The listing builds one solid part. Answer for the finished solid, in the listing's coordinates (mm). A direction names the side the tool comes from. Coordinates: 2 decimals unless noted, no trailing zeros. Return JSON: item names as keys, results as strings. Group by question number.
1. Which of the six approach directions +Z, -Z, +X, -X, +Y, -Y give full straight-line access (tool end or side, diameter ignored) to faces 4 (the face through (-22.23, 10.37, -10.32)), 5 (the face through (-33.142, 10.018, -8.724))?
2. Each of these flat-tipped pins is pushed along its axis until it touches: P1, Ø1.5, axis at y = 6.5, z = -7.5, coming from the +X side; P2, Ø4.5, axis at x = -26.99, y = 10.16, coming from the +Z side; P3, Ø12.5, axis at x = -17.46, z = 0, coming from the -Y side; P4, Ø1, axis at x = -7.5, z = -9, coming from the -Y side. Where does it stop, or does it pass through?
3. Section A-A (z = 0) is taken. State how many separate pieces and enclosed holes the cut face has, and give its area (3 significant figures).
4. Find the intervals of material crossed by line 1 along X through (y, z) = (6, -10); line 2 along Z through (x, y) = (-28, 13.75); line 3 along X through (y, z) = (10.16, -10.7) (3 decimals), in increasing order.
5. The mould has two halves that part along Z. Classify faces 1 (the face through (-10, 8, -7.874)), 2 (the face through (-34.925, 10, 3)), 3 (the face through (-22.22, 10.15, 0.21)): pulls with the +Z half, pulls with the -Z half, needs draft (parallel to the pull), parting line crosses it, or undercut.
```python
from build123d import *

# Parameters (mm, degrees)
BOSS_EXTRUDE1_DEPTH                             = 10.16
BOSS_EXTRUDE1_DEPTH_BACK                        = 12.7
SKETCH2_W                                       = 34.925
SKETCH2_H                                       = 20.32
SKETCH2_R                                       = 2.4892
SKETCH3_R                                       = 4.7625
CUT_EXTRUDE1_DEPTH                              = 43.35502361
CBORE_FOR_10_SOCKET_HEAD_CAP_SCREW1_D           = 4.9784
CBORE_FOR_10_SOCKET_HEAD_CAP_SCREW1_CBORE_D     = 9.525
CBORE_FOR_10_SOCKET_HEAD_CAP_SCREW1_CBORE_DEPTH = 4.826
FILLET1_R                                       = 9.525


with BuildPart() as part:
    # Sketch2 → Boss-Extrude1 (new, two sides: drawn at the far end of the back side and taken through both)
    with BuildSketch(Plane.XY.offset(-BOSS_EXTRUDE1_DEPTH_BACK)):
        with Locations((-17.4625, 10.16)):
            Rectangle(SKETCH2_W, SKETCH2_H)
        with Locations((-7.9375, 10.16)):
            Circle(SKETCH2_R, mode=Mode.SUBTRACT)
        with Locations((-26.9875, 10.16)):
            Circle(SKETCH2_R, mode=Mode.SUBTRACT)
    extrude(amount=BOSS_EXTRUDE1_DEPTH + BOSS_EXTRUDE1_DEPTH_BACK)

    # Sketch3 → Cut-Extrude1 (cut, through all)
    with BuildSketch(Plane.XZ):
        with Locations((-17.4625, 0)):
            Circle(SKETCH3_R)
    extrude(amount=-CUT_EXTRUDE1_DEPTH, mode=Mode.SUBTRACT)

    # Sketch4 → Cut-Revolve1 (revolve, cut)
    with BuildSketch(Plane.XY, mode=Mode.PRIVATE) as cut_revolve1_sk:
        with BuildLine():
            Line((-31.75, 20.32), (-17.4625, 20.32))
            Line((-17.4625, 20.32), (-17.4625, 0))
            Line((-17.4625, 0), (-31.75, 0))
            ThreePointArc((-31.75, 0), (-25.014807909, 2.789807909), (-22.225, 9.525))
            Line((-22.225, 9.525), (-22.225, 10.795))
            ThreePointArc((-22.225, 10.795), (-25.014807909, 17.530192091), (-31.75, 20.32))
        make_face()
    revolve(cut_revolve1_sk.sketch.rotate(Axis((-17.4625, 20.32, 0), (0, -1, 0)), 270), axis=Axis((-17.4625, 20.32, 0), (0, -1, 0)), mode=Mode.SUBTRACT)

    # CBORE for #10 Socket Head Cap Screw1 (through all)
    with Locations(Plane(origin=(0, 0, -12.7), x_dir=(-1, 0, 0), z_dir=(0, 0, -1))):
        with Locations((26.9875, 10.16), (7.9375, 10.16)):
            CounterBoreHole(CBORE_FOR_10_SOCKET_HEAD_CAP_SCREW1_D / 2, CBORE_FOR_10_SOCKET_HEAD_CAP_SCREW1_CBORE_D / 2, CBORE_FOR_10_SOCKET_HEAD_CAP_SCREW1_CBORE_DEPTH)

    # Fillet1
    # the kernel refuses this fillet: 9.525 mm, written as the material it takes off along each edge
    with BuildSketch(Plane(origin=(-34.925, -23.8125, -12.7), x_dir=(1, 0, 0), z_dir=(0, 1, 0))) as fillet1_piece_1:
        with BuildLine():
            CenterArc((FILLET1_R, -FILLET1_R), FILLET1_R, 90, 90)
            Line((0, -FILLET1_R), (0, 0))
            Line((0, 0), (FILLET1_R, 0))
        make_face()
    extrude(amount=67.945, mode=Mode.SUBTRACT)
    with BuildSketch(Plane(origin=(0, 44.1325, -12.7), x_dir=(0, 0, 1), z_dir=(0, -1, 0))) as fillet1_piece_2:
        with BuildLine():
            CenterArc((FILLET1_R, FILLET1_R), FILLET1_R, 180, 90)
            Line((0, FILLET1_R), (0, 0))
            Line((0, 0), (FILLET1_R, 0))
        make_face()
    extrude(amount=67.945, mode=Mode.SUBTRACT)


solid = part.part
```
The answers:
{
 "1": {"face 4": "-Z", "face 5": "-Z, -X, +Y, -Y"},
 "2": {"P1": "stops at x = -0.7", "P2": "passes through", "P3": "stops at y = 4.41", "P4": "stops at y = 0.01"},
 "3": {"separate pieces": "2", "enclosed holes": "2", "area": "399 mm2"},
 "4": {"line 1": "x = -32.04 to -29.31, -24.67 to -10.26, -5.62 to -2.88", "line 2": "z = -7.87 to 10.16", "line 3": "x = -22.225 to -12.7"},
 "5": {"face 1": "pulls with the -Z half", "face 2": "needs draft", "face 3": "undercut"}
}
